The model under review builds one solid part; all positions refer to its coordinate system, in mm. Face numbers are marked on the shaded views. A direction names the side the tool comes from. Round coordinates to 2 decimals unless told otherwise and drop trailing zeros. Loops run counter-clockwise (first coordinate to the right, second up) from the corner with the lowest first, then second, coordinate; pieces in that order, holes last. Notation, with made-up numbers: (34, -20) -> (47, -20) arc R20 cw to (47, 16) -> close; hole circle Ø3 at (40, 67.25). An arc over 180 degrees is marked (long way). Use a Markdown table: item, result. Add a question column.
1) Consider section A-A on z = 0. State how many separate pieces and enclosed holes the cut face has, plus the area to 3 significant figures.
2) Wall thickness on probe 1 along Y at (x, z) = (-3.5, 26); probe 2 along Z at (x, y) = (0, -28.75); probe 3 along Z at (x, y) = (58.5, 1.5): over which ranges is each line inside the solid? List them lowest first.
3) Consider section C-C on x = 130. Give the boundary of the cut face in (y, z), plus the area to 3 significant figures.
4) Mouldability with a two-part tool opening along X and no side actions: class the marked faces 1, 2 and 3 as released by +X, released by -X, zero draft, split by the parting line, or undercut.
5) Insertion check: pin 1 (24 mm diameter, centred on x = 91.5, y = 0.5, fed in from +Z); pin 2 (4 mm diameter, centred on y = -14.5, z = 15.5, fed in from +X); pin 3 (4 mm diameter, centred on y = -15.5, z = -12.5, fed in from +X). Each pin has a flat end and moves straight along its axis. Give the tip position at first contact, or say it passes through.
6) Consider section D-D on y = 0. Give the boundary of the cut face in (x, z), plus the area to 3 significant figures.
7) For the marked faces 4, 5, 6, 7 and 8, list the 3-axis set-ups (+Z, -Z, +X, -X, +Y, -Y) from which the entire face can be reached by the end or side of a thin tool; tool diameter is ignored.
8) Consider section B-B on x = 0. Give the boundary of the cut face in (y, z).
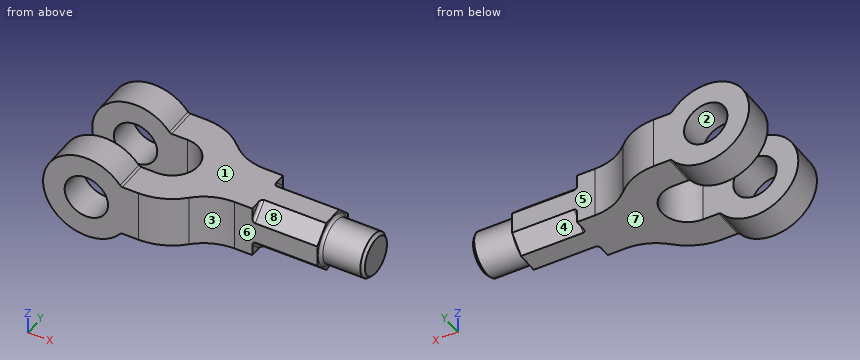
Autodesk Inventor part; units mm, degrees
ref_plane "YZ Plane" through (0, 0, 0) normal (1, 0, 0) x (0, 1, 0)
ref_plane "XZ Plane" through (0, 0, 0) normal (0, 1, 0) x (-1, 0, 0)
ref_plane "XY Plane" through (0, 0, 0) normal (0, 0, 1) x (1, 0, 0)
sketch "Sketch2" plane through (0, 0, 0) normal (0, 0, 1) x (1, 0, 0)
  line L0 (0, 18) -> (36, 18)
  line L1 (36, -18) -> (0, -18)
  arc A0 (36, -18) -> (36, 18) centre (36, 0) ccw
  line L2 (0, 40) -> (36, 40)
  line L3 (36, -40) -> (0, -40)
  line L4 (0, 40) -> (0, 18)
  line L5 (0, -18) -> (0, -40)
  line L6 (89.479, 18) -> (147, 18)
  line L7 (147, 18) -> (147, -18)
  line L8 (147, -18) -> (89.479, -18)
  arc A1 (36, -40) -> (64.1468, -28.4211) centre (36, 0) ccw
  arc A2 (64.1468, 28.4211) -> (36, 40) centre (36, 0) ccw
  line L9 (0, 75.6) -> (0, -75.6)
  arc A3 (64.1468, 28.4211) -> (89.479, 18) centre (89.479, 54) ccw
  arc A4 (89.479, -18) -> (64.1468, -28.4211) centre (89.479, -54) ccw
  point P0 (0, 0)
  point P1 (0, 0)
  point P2 (71.7211, 18)
  point P3 (71.7211, -18)
  dimension "d3" = 147
  dimension "d4" = 36
  dimension "d5" = 18
  dimension "d6" = 36
extrude "Extrusion1" add sketch "Sketch2" along normal mid plane 36 contours L4 L2 A2 A3 L6 L7 L8 A4 A1 L3 L5 L1 A0 L0
sketch "Sketch3" plane through (0, 40, 18) normal (0, 1, 0) x (1, 0, 0)
  circle A0 centre (0, 18) radius 30
  dimension "d11" = 60
extrude "Extrusion2" add sketch "Sketch3" against normal blind 22
sketch "Sketch4" plane through (36, 40, 18) normal (0, 1, 0) x (1, 0, 0)
  circle A0 centre (-36, 18) radius 15
  dimension "d14" = 30
extrude "Extrusion3" cut sketch "Sketch4" against normal blind 22
mirror "Mirror1" about plane through (0, 0, 0) normal (0, 1, 0) of "Extrusion3", "Extrusion2"
sketch "Sketch5" plane through (147, -18, 18) normal (1, 0, 0) x (0, 0, -1)
  line L0 (36, 36) -> (36, 0)
  line L1 (36, 10.5442) -> (25.4558, 0)
  line L2 (25.4558, 0) -> (10.5442, 0)
  line L3 (10.5442, 0) -> (0, 10.5442)
  line L4 (0, 10.5442) -> (0, 25.4558)
  line L5 (0, 25.4558) -> (10.5442, 36)
  line L6 (10.5442, 36) -> (25.4558, 36)
  line L7 (25.4558, 36) -> (36, 25.4558)
  line L8 (36, 25.4558) -> (36, 10.5442)
  line L9 (36, 36) -> (0, 36)
  line L10 (0, 0) -> (0, 36)
  line L11 (36, 0) -> (0, 0)
  line L12 (36, 36) -> (36, 0)
  point P0 (18, 18)
  point P1 (18, 18)
  point P2 (36, 18)
  point P3 (36, 36)
  point P4 (36, 0)
extrude "Extrusion4" cut sketch "Sketch5" against normal blind 45 contours L0 L7 L9 | L0 L11 L1 | L5 L10 L9 | L11 L10 L3
sketch "Sketch6" plane through (147, -7.4558, 18) normal (1, 0, 0) x (0, 0, -1)
  circle A0 centre (18, 7.4558) radius 15
  dimension "d19" = 30
extrude "Extrusion5" add sketch "Sketch6" along normal blind 30
fillet "Fillet1" radius 2 9 edges at (24, 29, 18) (24, -29, 18) (102, 12.7279, 12.7279) (147, 0, 15) (24, 29, -18) (24, -29, -18) (102, 12.7279, -12.7279) (102, -12.7279, -12.7279) (102, -12.7279, 12.7279)
chamfer "Chamfer1" distance 2 angle 45 1 edges at (177, 0, 15)
properties part number "fork end"
Result set:
| question | item | result |
|---|---|---|
| 1 | separate pieces | 3 |
| 1 | enclosed holes | 0 |
| 1 | area | 7,170 mm2 |
| 2 | probe 1 | -40 to -18, 18 to 40 |
| 2 | probe 2 | -30 to -15, 15 to 30 |
| 2 | probe 3 | -18 to 18 |
| 3 | outline | (-18, -7.46) -> (-7.46, -18) -> (7.46, -18) -> (18, -7.46) -> (18, 7.46) -> (7.46, 18) -> (-7.46, 18) -> (-18, 7.46) -> close |
| 3 | area | 1,070 mm2 |
| 4 | face 1 | zero draft |
| 4 | face 2 | undercut |
| 4 | face 3 | released by +X |
| 5 | pin 1 | z = 18 |
| 5 | pin 2 | x = 102.16 |
| 5 | pin 3 | x = 147 |
| 6 | outline | (54, -18) -> (147, -18) -> (147, -17) arc R2 cw to (149, -15) -> (175, -15) -> (177, -13) -> (177, 13) -> (175, 15) -> (149, 15) arc R2 cw to (147, 17) -> (147, 18) -> (54, 18) -> close |
| 6 | area | 4,250 mm2 |
| 7 | face 4 | -Z, +X, +Y |
| 7 | face 5 | +Z, -Z, +X, +Y |
| 7 | face 6 | +Z, -Z, +X, -Y |
| 7 | face 7 | -Z, +X, +Y, -Y |
| 7 | face 8 | +Z, +X, -Y |
| 8 | outline | (-40, -30) -> (-18, -30) -> (-18, -15) -> (-40, -15) -> close; (-40, 15) -> (-18, 15) -> (-18, 30) -> (-40, 30) -> close; (18, -30) -> (40, -30) -> (40, -15) -> (18, -15) -> close; (18, 15) -> (40, 15) -> (40, 30) -> (18, 30) -> close |
